The model under review builds one solid part; all positions refer to its coordinate system, in mm. A direction names the side the tool comes from. Round coordinates to 2 decimals unless told otherwise and drop trailing zeros. Loops run counter-clockwise (first coordinate to the right, second up) from the corner with the lowest first, then second, coordinate; pieces in that order, holes last. Notation, with made-up numbers: (-32, 37) -> (-23, 37) arc R19 cw to (-23, 48) -> close; hole circle Ø5 at (88, 8.5). An arc over 180 degrees is marked (long way). Use a Markdown table: item, result. Add a question column.
1) Consider section A-A on y = 6. Give the boundary of the cut face in (x, z), plus the area to 3 significant figures.
2) Consider section B-B on x = 0. Give the boundary of the cut face in (y, z).
3) For faces 1 (the flat face through (3, 3, 9.7)), 2 (the cylindrical face through (5.25, 6.03, -1.43)), list the 3-axis set-ups (+Z, -Z, +X, -X, +Y, -Y) from which the entire face can be reached by the end or side of a thin tool; tool diameter is ignored.
4) Consider section C-C on x = 1.5. Give the boundary of the cut face in (y, z), plus the area to 3 significant figures.
5) Wall thickness on probe 1 along Z at (x, y) = (8, 1.75); probe 2 along Y at (x, z) = (6, -0.5); probe 3 along Y at (x, z) = (8, 8): over which ranges is each line inside the solid? List them lowest first.
from build123d import *

# Parameters (mm, degrees)
SKETCH_W     = 11.5
SKETCH_H     = 11.5
PAD_DEPTH    = 9.6
FILLET_R     = 1.5
SKETCH001_R  = 0.75
PAD001_DEPTH = 3.5


with BuildPart() as fillet_body:
    # Sketch → Pad (new body)
    with BuildSketch(Plane.XY.offset(0.1)):
        with Locations((3, 3)):
            Rectangle(SKETCH_W, SKETCH_H)
    extrude(amount=PAD_DEPTH)

    # Fillet
    fillet_edges = [fillet_body.edges().sort_by_distance(p)[0] for p in [
        (8.75, -2.75, 4.9),
        (8.75, 8.75, 4.9),
        (-2.75, -2.75, 4.9),
        (-2.75, 8.75, 4.9),
    ]]
    fillet(fillet_edges, radius=FILLET_R)


with BuildPart() as obj1:
    # Sketch001 → Pad001 (new body)
    with BuildSketch(Plane.XY.offset(0.5)):
        Circle(SKETCH001_R)
        with Locations((6, 6)):
            Circle(SKETCH001_R)
    extrude(amount=-PAD001_DEPTH)

    # obj1: union Fillet body
    add(fillet_body.part)


solid = obj1.part
Result set:
| question | item | result |
|---|---|---|
| 1 | outline | (-2.75, 0.1) -> (5.25, 0.1) -> (5.25, -3) -> (6.75, -3) -> (6.75, 0.1) -> (8.75, 0.1) -> (8.75, 9.7) -> (-2.75, 9.7) -> close |
| 1 | area | 115 mm2 |
| 2 | outline | (-2.75, 0.1) -> (-0.75, 0.1) -> (-0.75, -3) -> (0.75, -3) -> (0.75, 0.1) -> (8.75, 0.1) -> (8.75, 9.7) -> (-2.75, 9.7) -> close |
| 3 | face 1 | +Z, +X, -X, +Y, -Y |
| 3 | face 2 | -Z |
| 4 | outline | (-2.75, 0.1) -> (8.75, 0.1) -> (8.75, 9.7) -> (-2.75, 9.7) -> close |
| 4 | area | 110 mm2 |
| 5 | probe 1 | 0.1 to 9.7 |
| 5 | probe 2 | 5.25 to 6.75 |
| 5 | probe 3 | -2.55 to 8.55 |
